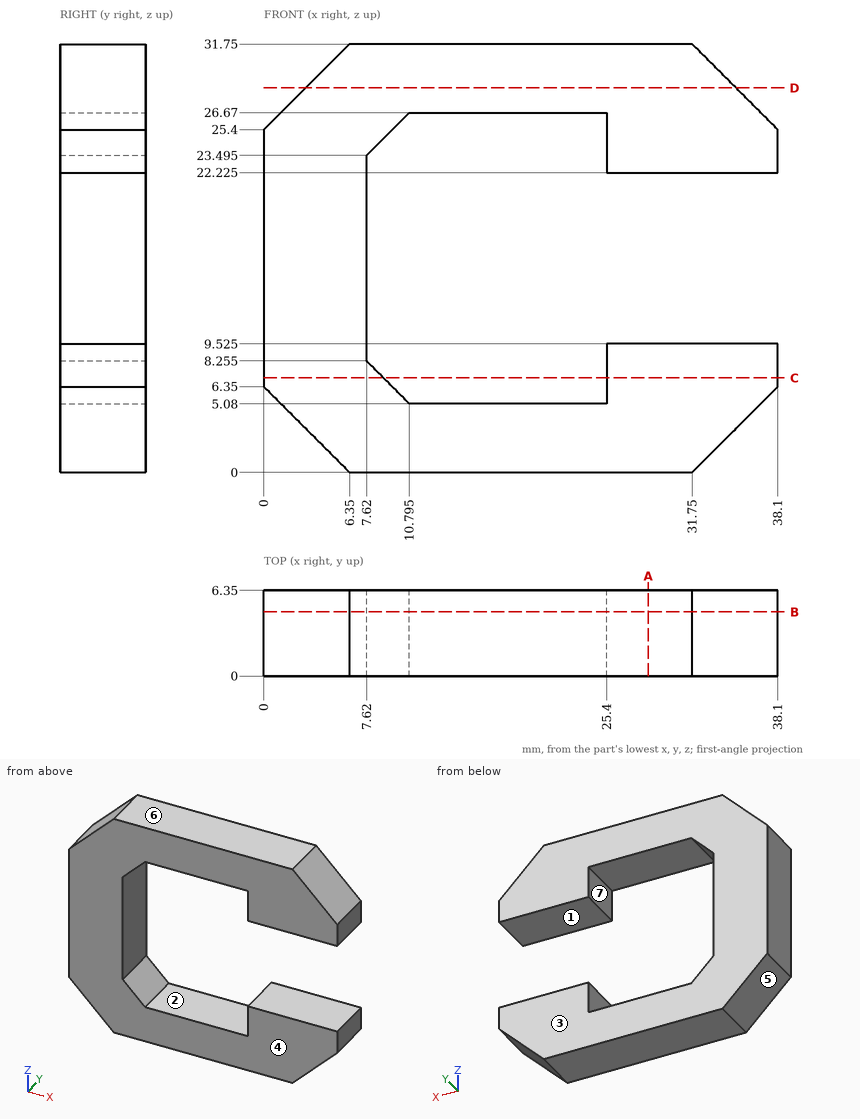
Geometry check sheet. Reference: drawing and pictorial views, mm from the part's lowest x, y, z. A direction names the side the tool comes from. Give positions to 0.01 mm unless a question says otherwise; leave off trailing zeros. Order: outer loops, then holes, each group sorted by start corner. A loop starts at its lowest first (then second) coordinate and runs counter-clockwise, first axis right, second up. Notation, with made-up numbers: M -17,5 L 41,5 A16 ccw 41,21 Z; hole C -18.75,84 d8. An arc over 180 degrees is marked long. Answer in a Markdown table with one row per item.
1) Cross-section at B-B, the plane y = 4.75. Enter the section's corners in (x, z) (3 decimals), plus the area to 3 significant figures.
Filled sheet:
| item | result |
|---|---|
| outline | M 0,6.35 L 6.35,0 L 31.75,0 L 38.1,6.35 L 38.1,9.525 L 25.4,9.525 L 25.4,5.08 L 10.795,5.08 L 7.62,8.255 L 7.62,23.495 L 10.795,26.67 L 25.4,26.67 L 25.4,22.225 L 38.1,22.225 L 38.1,25.4 L 31.75,31.75 L 6.35,31.75 L 0,25.4 Z |
| area | 594 mm2 |
2) Cross-section at A-A, the plane x = 28.5. Enter the section's corners in (y, z) (3 decimals).
Filled sheet:
| item | result |
|---|---|
| outline | M 0,0 L 6.35,0 L 6.35,9.525 L 0,9.525 Z; M 0,22.225 L 6.35,22.225 L 6.35,31.75 L 0,31.75 Z |
3) Thickness scan on L1, parallel to Z at x = 11, y = 3.75; L2, parallel to Z at x = 27, y = 3.25 (3 decimals); L3, parallel to X at y = 3.25, z = 19.5. Record the ranges inside material, lowest first. Write a range as [from, to].
Filled sheet:
| item | result |
|---|---|
| L1 | z = [0, 5.08], [26.67, 31.75] |
| L2 | z = [0, 9.525], [22.225, 31.75] |
| L3 | x = [0, 7.62] |
4) Cross-section at C-C, the plane z = 7. Enter the section's corners in (x, y) (3 decimals).
Filled sheet:
| item | result |
|---|---|
| outline | M 0,0 L 8.875,0 L 8.875,6.35 L 0,6.35 Z; M 25.4,0 L 38.1,0 L 38.1,6.35 L 25.4,6.35 Z |
5) Gauge pin test, flat ends, axial feed: P1, Ø8, axis at x = 12.5, z = 5.5, coming from the +Y side; P2, Ø1.9, axis at y = 2, z = 18.5, coming from the +X side. Record the tip position at first contact, or that the pin passes through.
Filled sheet:
| item | result |
|---|---|
| P1 | stops at y = 6.35 |
| P2 | stops at x = 7.62 |
6) Cross-section at D-D, the plane z = 28.5. Enter the section's corners in (x, y).
Filled sheet:
| item | result |
|---|---|
| outline | M 3.1,0 L 35,0 L 35,6.35 L 3.1,6.35 Z |
7) Release check for a two-part mould opening along Z. For the marked faces 4, 5, 6 and 7 record: +Z half, -Z half, draft (parallel to the pull), parting line (faces both ways), or undercut.
Filled sheet:
| item | result |
|---|---|
| face 4 | draft |
| face 5 | -Z half |
| face 6 | +Z half |
| face 7 | undercut |
8) Access from +Z, -Z, +X, -X, +Y, -Y to the whole of each face (thin tool, end or side, straight path). Record for the marked faces 1, 2 and 3.
Filled sheet:
| item | result |
|---|---|
| face 1 | +X, +Y, -Y |
| face 2 | +Y, -Y |
| face 3 | +Z, -Z, +X, -X, +Y |
